```python
from build123d import *

# Parameters (mm, degrees)
BOSS_EXTRUDE1_DEPTH = 23
CUT_EXTRUDE1_START  = -54
CUT_EXTRUDE1_DEPTH  = 54
CUT_EXTRUDE2_REACH  = 128.369
SKETCH3_R           = 6
SKETCH3_3_W         = 28
SKETCH3_3_H         = 28
SKETCH3_3_R         = 6
CUT_EXTRUDE3_DEPTH  = 12
SKETCH3_4_W         = 195
SKETCH3_4_H         = 35
SKETCH3_4_W_2       = 28
SKETCH3_4_H_2       = 28
CUT_EXTRUDE4_DEPTH  = 2
FILLET1_R           = 8
CHAMFER1_SIZE       = 2
CHAMFER2_SIZE       = 1
SKETCH4_R           = 4
CUT_EXTRUDE5_DEPTH  = 52


# Read off the part's stored shape, not the designer's step: Cut-Extrude1
with BuildPart() as part:
    # Sketch1 → Boss-Extrude1 (new, symmetric)
    with BuildSketch(Plane.XY):
        with BuildLine():
            Line((-104, 0), (104, 0))
            Line((104, 0), (99.985564599, 14))
            Line((99.985564599, 14), (54, 14))
            Line((54, 14), (54, 68))
            Line((54, 68), (28, 68))
            Line((28, 68), (28, 52))
            Line((28, 52), (24, 52))
            Line((24, 52), (24, 48))
            ThreePointArc((24, 48), (0, 24), (-24, 48))
            Line((-24, 48), (-24, 52))
            Line((-24, 52), (-28, 52))
            Line((-28, 52), (-28, 68))
            Line((-28, 68), (-54, 68))
            Line((-54, 68), (-54, 14))
            Line((-54, 14), (-99.985564599, 14))
            Line((-99.985564599, 14), (-104, 0))
        make_face()
    extrude(amount=BOSS_EXTRUDE1_DEPTH, both=True)

    # Cut-Extrude1 outline → Cut-Extrude1 (cut)
    with BuildSketch(Plane(origin=(0, 68, 0), x_dir=(1, 0, 0), z_dir=(0, 1, 0)).offset(CUT_EXTRUDE1_START)):
        with BuildLine():
            ThreePointArc((-54, 0), (-52.698550436, 11.784005345), (-48.856934001, 23))
            Line((-48.856934001, 23), (-54, 23))
            Line((-54, 23), (-54, 0))
        make_face()
        with BuildLine():
            ThreePointArc((-48.856934001, -23), (-52.698550436, -11.784005345), (-54, 0))
            Line((-54, 0), (-54, -23))
            Line((-54, -23), (-48.856934001, -23))
        make_face()
        with BuildLine():
            Line((54, 23), (48.856934001, 23))
            ThreePointArc((48.856934001, 23), (52.698550436, 11.784005345), (54, 0))
            Line((54, 0), (54, 23))
        make_face()
        with BuildLine():
            Line((54, -23), (54, 0))
            ThreePointArc((54, 0), (52.698550436, -11.784005345), (48.856934001, -23))
            Line((48.856934001, -23), (54, -23))
        make_face()
    extrude(amount=CUT_EXTRUDE1_DEPTH, mode=Mode.SUBTRACT)

    # Sketch3 → Cut-Extrude2 (cut, up to next)
    with BuildSketch(Plane.XZ, mode=Mode.PRIVATE) as cut_extrude2_sk1:
        with Locations(Location((-39, 0, 0), (0, 0, 270))):
            Circle(SKETCH3_R)
    cut_extrude2_tool1 = extrude(cut_extrude2_sk1.sketch, amount=-CUT_EXTRUDE2_REACH, mode=Mode.PRIVATE) & part.part
    # Sketch3 → Cut-Extrude2 (cut, up to next)
    with BuildSketch(Plane.XZ, mode=Mode.PRIVATE) as cut_extrude2_sk2:
        with Locations(Location((39, 0, 0), (0, 0, 270))):
            Circle(SKETCH3_R)
    cut_extrude2_tool2 = extrude(cut_extrude2_sk2.sketch, amount=-CUT_EXTRUDE2_REACH, mode=Mode.PRIVATE) & part.part
    # Sketch3 → Cut-Extrude2 (cut, up to next)
    with BuildSketch(Plane.XZ, mode=Mode.PRIVATE) as cut_extrude2_sk3:
        with BuildLine():
            Line((77, -6), (85, -6))
            ThreePointArc((85, -6), (91, 0), (85, 6))
            Line((85, 6), (77, 6))
            ThreePointArc((77, 6), (71, 0), (77, -6))
        make_face()
    cut_extrude2_tool3 = extrude(cut_extrude2_sk3.sketch, amount=-CUT_EXTRUDE2_REACH, mode=Mode.PRIVATE) & part.part
    # Sketch3 → Cut-Extrude2 (cut, up to next)
    with BuildSketch(Plane.XZ, mode=Mode.PRIVATE) as cut_extrude2_sk4:
        with BuildLine():
            ThreePointArc((-85, -6), (-91, 0), (-85, 6))
            Line((-85, 6), (-77, 6))
            ThreePointArc((-77, 6), (-71, 0), (-77, -6))
            Line((-77, -6), (-85, -6))
        make_face()
    cut_extrude2_tool4 = extrude(cut_extrude2_sk4.sketch, amount=-CUT_EXTRUDE2_REACH, mode=Mode.PRIVATE) & part.part
    add(cut_extrude2_tool1.solids().sort_by_distance((-39, 0, 0))[0], mode=Mode.SUBTRACT)
    add(cut_extrude2_tool2.solids().sort_by_distance((39, 0, 0))[0], mode=Mode.SUBTRACT)
    add(cut_extrude2_tool3.solids().sort_by_distance((81, 0, 0))[0], mode=Mode.SUBTRACT)
    add(cut_extrude2_tool4.solids().sort_by_distance((-81, 0, 0))[0], mode=Mode.SUBTRACT)

    # Sketch3<3> → Cut-Extrude3 (cut)
    # profile 1 of 2: a face of its own
    with BuildSketch(Plane.XZ):
        with Locations((39, 0)):
            Rectangle(SKETCH3_3_W, SKETCH3_3_H)
        with Locations(Location((39, 0, 0), (0, 0, 270))):
            Circle(SKETCH3_3_R, mode=Mode.SUBTRACT)
    # profile 2 of 2: a face of its own
    with BuildSketch(Plane.XZ):
        with Locations((-39, 0)):
            Rectangle(SKETCH3_3_W, SKETCH3_3_H)
        with Locations(Location((-39, 0, 0), (0, 0, 270))):
            Circle(SKETCH3_3_R, mode=Mode.SUBTRACT)
    extrude(amount=-CUT_EXTRUDE3_DEPTH, mode=Mode.SUBTRACT)

    # Sketch3<4> → Cut-Extrude4 (cut)
    with BuildSketch(Plane.XZ):
        Rectangle(SKETCH3_4_W, SKETCH3_4_H)
        with BuildLine():
            ThreePointArc((85, -6), (91, 0), (85, 6))
            Line((85, 6), (77, 6))
            ThreePointArc((77, 6), (71, 0), (77, -6))
            Line((77, -6), (85, -6))
        make_face(mode=Mode.SUBTRACT)
        with Locations((-39, 0)):
            Rectangle(SKETCH3_4_W_2, SKETCH3_4_H_2, mode=Mode.SUBTRACT)
        with Locations((39, 0)):
            Rectangle(SKETCH3_4_W_2, SKETCH3_4_H_2, mode=Mode.SUBTRACT)
        with BuildLine():
            Line((-77, -6), (-85, -6))
            ThreePointArc((-85, -6), (-91, 0), (-85, 6))
            Line((-85, 6), (-77, 6))
            ThreePointArc((-77, 6), (-71, 0), (-77, -6))
        make_face(mode=Mode.SUBTRACT)
    extrude(amount=-CUT_EXTRUDE4_DEPTH, mode=Mode.SUBTRACT)

    # Fillet1
    fillet1_edges = [part.edges().sort_by_distance(p)[0] for p in [
        (-52.698550436, 14, -11.784005345),
        (52.698550436, 14, -11.784005345),
    ]]
    fillet(fillet1_edges, radius=FILLET1_R)

    # Chamfer1
    chamfer1_edges = [part.edges().sort_by_distance(p)[0] for p in [
        (-24, 50, -23),
        (0, 24, -23),
        (24, 50, -23),
        (24, 50, 23),
        (0, 24, 23),
        (-24, 50, 23),
    ]]
    chamfer(chamfer1_edges, length=CHAMFER1_SIZE)

    # Chamfer2
    chamfer2_edges = [part.edges().sort_by_distance(p)[0] for p in [
        (91, 14, 0),
        (81, 14, -6),
        (71, 14, 0),
        (-91, 14, 0),
        (-71, 14, 0),
        (-81, 14, -6),
        (-81, 14, 6),
        (81, 14, 6),
    ]]
    chamfer(chamfer2_edges, length=CHAMFER2_SIZE)

    # Sketch4 → Cut-Extrude5 (cut)
    with BuildSketch(Plane(origin=(0, 68, 0), x_dir=(1, 0, 0), z_dir=(0, 1, 0))):
        with Locations(Location((0, 0, 0), (0, 0, 180))):
            Circle(SKETCH4_R)
    extrude(amount=-CUT_EXTRUDE5_DEPTH, mode=Mode.SUBTRACT)


solid = part.part
```
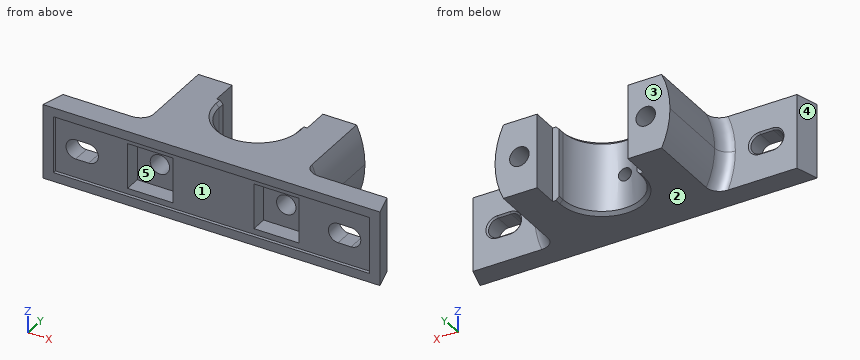
Design review of the part built by this model. Coordinates are the model's own, in mm. Face numbers are marked on the shaded views. A direction names the side the tool comes from. Coordinates: 2 decimals unless noted, no trailing zeros. Loops run counter-clockwise (first coordinate to the right, second up) from the corner with the lowest first, then second, coordinate; pieces in that order, holes last. Notation, with made-up numbers: (-12, -6) -> (6, -6) arc R21 cw to (6, 19) -> close; hole circle Ø10 at (80, 77.25). An arc over 180 degrees is marked (long way). Answer as a JSON object with one key per item and string values.
Q1. Take a section at C-C on x = 43. Give the boundary of the cut face in (y, z), plus the area to 3 significant figures.
Answer block:
{"outline": "(0, -23) -> (68, -23) -> (68, -4.47) -> (12, -4.47) -> (12, -14) -> (2, -14) -> (2, -17.5) -> (0, -17.5) -> close; (0, 17.5) -> (2, 17.5) -> (2, 14) -> (12, 14) -> (12, 4.47) -> (68, 4.47) -> (68, 23) -> (0, 23) -> close", "area": "2,280 mm^2"}
Q2. Tool access review of the marked faces 1 and 2: name each direction out of +Z, -Z, +X, -X, +Y, -Y from which nothing blocks a thin tool from reaching the whole face with its end or side.
Answer block:
{"face 1": "-Y", "face 2": "-Z, +X, -X, +Y, -Y"}
Q3. Take a section at D-D on y = 38.5. Give the number of separate pieces and of enclosed holes in the cut face, plus the area to 3 significant figures.
Answer block:
{"separate pieces": "2", "enclosed holes": "2", "area": "2,550 mm^2"}
Q4. The part is to be moulded in two halves that separate along X. For the marked faces 3, 4 and 5, say which applies: +X half, -X half, draft (parallel to the pull), parting line (faces both ways), or undercut.
Answer block:
{"face 3": "draft", "face 4": "-X half", "face 5": "undercut"}
Q5. Take a section at B-B on y = 8. Give the boundary of the cut face in (x, z).
Answer block:
{"outline": "(-101.71, -23) -> (101.71, -23) -> (101.71, 23) -> (-101.71, 23) -> close; hole (-85, -6) -> (-77, -6) arc R6 ccw to (-77, 6) -> (-85, 6) arc R6 ccw to start; hole (-53, -14) -> (-25, -14) -> (-25, 14) -> (-53, 14) -> close; hole (25, -14) -> (53, -14) -> (53, 14) -> (25, 14) -> close; hole (77, -6) -> (85, -6) arc R6 ccw to (85, 6) -> (77, 6) arc R6 ccw to start"}
Q6. Clearance check with flat-ended pins moving along their axes: pin 1 Ø8 at (y, z) = (9.5, -2) entering from +X; pin 2 Ø21 at (x, z) = (-75, -5.5) entering from +Y; pin 3 Ø2 at (y, z) = (50, 3.5) entering from -X; pin 4 Ø7 at (x, z) = (39, 0) entering from -Y. State where each tip first meets the part, or that it passes through.
Answer block:
{"pin 1": "stops at x = 102.42", "pin 2": "stops at y = 14", "pin 3": "stops at x = -53.94", "pin 4": "passes through"}
Q7. To check wall thickness, follow L1, parallel to X at y = 53.5, z = 0; L2, parallel to X at y = 58, z = 2.5; L3, parallel to Z at x = 0, y = 19. State the ranges of each line that lie inside material, in increasing order.
Answer block:
{"L1": "x = -54 to -45, -33 to -28, 28 to 33, 45 to 54", "L2": "x = -53.94 to -44.45, -33.55 to -28, 28 to 33.55, 44.45 to 53.94", "L3": "z = -23 to -4, 4 to 23"}
Q8. Take a section at A-A on y = 59.5. Give the boundary of the cut face in (x, z), plus the area to 3 significant figures.
Answer block:
{"outline": "(-48.86, -23) -> (-28, -23) -> (-28, 23) -> (-48.86, 23) arc R54 ccw to start; (28, -23) -> (48.86, -23) arc R54 ccw to (48.86, 23) -> (28, 23) -> close; hole circle Ø12 at (-39, 0); hole circle Ø12 at (39, 0)", "area": "2,010 mm^2"}
